The listing builds one solid part. Answer for the finished solid, in the listing's coordinates (mm). Face numbers are marked on the shaded views. Coordinates: 2 decimals unless noted, no trailing zeros. Loops run counter-clockwise (first coordinate to the right, second up) from the corner with the lowest first, then second, coordinate; pieces in that order, holes last. Notation, with made-up numbers: (22, 67.25) - (66, 67.25) arc R21 ccw to (66, 101.25) - close; hole circle Ø8 at (-32, 44). An arc over 180 degrees is marked (long way). Use one line per item in the form item = value. Start each with the question number.
```python
from build123d import *

# Parameters (mm, degrees)
SKETCH1_W           = 45
SKETCH1_H           = 15
SKETCH1_R           = 2
BOSS_EXTRUDE1_DEPTH = 6
FILLET1_R           = 4


with BuildPart() as part:
    # Sketch1 → Boss-Extrude1 (new body)
    with BuildSketch(Plane.XY):
        with Locations((12.5, 0)):
            Rectangle(SKETCH1_W, SKETCH1_H)
        Circle(SKETCH1_R, mode=Mode.SUBTRACT)
        with Locations((25, 0)):
            Circle(SKETCH1_R, mode=Mode.SUBTRACT)
    extrude(amount=BOSS_EXTRUDE1_DEPTH)

    # Fillet1
    fillet1_edges = [part.edges().sort_by_distance(p)[0] for p in [
        (-10, 7.5, 3),
        (35, 7.5, 3),
        (35, -7.5, 3),
        (-10, -7.5, 3),
    ]]
    fillet(fillet1_edges, radius=FILLET1_R)


solid = part.part
```
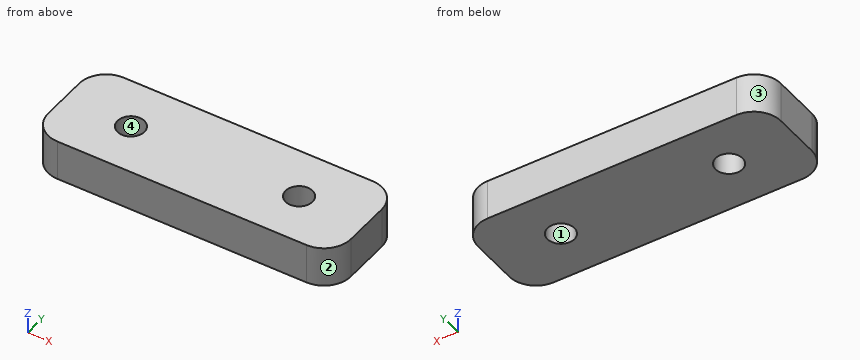
(1) A cutting plane is placed at D-D (x = 24). Determine the outline of the cut face in (y, z).
(2) A cutting plane is placed at B-B (x = 0). Determine the outline of the cut face in (y, z), then the cut area to 3 significant figures.
(3) Determine the mould class of the marked faces 1, 2, 3 and 4 for opening direction Y: +Y half, -Y half, draft (parallel to the pull), parting line (faces both ways), or undercut.
(4) A cutting plane is placed at A-A (y = 0). Determine the outline of the cut face in (x, z).
(5) A cutting plane is placed at C-C (z = 0.5). Determine the outline of the cut face in (x, y).
(6) Find the intervals of material crossed by probe 1 along Y at (x, z) = (0, 2.35); probe 2 along X at (y, z) = (1.75, 1.05); probe 3 along X at (y, z) = (0.5, 3.75), in increasing order. Write a range as from..to.
Evaluation:
q1.outline = (-7.5, 0) - (-1.73, 0) - (-1.73, 6) - (-7.5, 6) - close; (1.73, 0) - (7.5, 0) - (7.5, 6) - (1.73, 6) - close
q2.outline = (-7.5, 0) - (-2, 0) - (-2, 6) - (-7.5, 6) - close; (2, 0) - (7.5, 0) - (7.5, 6) - (2, 6) - close
q2.area = 66.0 mm^2
q3.face_1 = undercut
q3.face_2 = -Y half
q3.face_3 = +Y half
q3.face_4 = undercut
q4.outline = (-10, 0) - (-2, 0) - (-2, 6) - (-10, 6) - close; (2, 0) - (23, 0) - (23, 6) - (2, 6) - close; (27, 0) - (35, 0) - (35, 6) - (27, 6) - close
q5.outline = (-10, -3.5) arc R4 ccw to (-6, -7.5) - (31, -7.5) arc R4 ccw to (35, -3.5) - (35, 3.5) arc R4 ccw to (31, 7.5) - (-6, 7.5) arc R4 ccw to (-10, 3.5) - close; hole circle Ø4 at (0, 0); hole circle Ø4 at (25, 0)
q6.probe_1 = -7.5..-2, 2..7.5
q6.probe_2 = -10..-0.97, 0.97..24.03, 25.97..35
q6.probe_3 = -10..-1.94, 1.94..23.06, 26.94..35
